```python
from build123d import *

# Parameters (mm, degrees)
F0_W     = 5
F0_H     = 4
F1_DEPTH = 6
F2_W     = 4
F2_H     = 2
F3_DEPTH = 25
F4_R     = 0.5
F5_DEPTH = 25
F6_R     = 1.25
F6_R_2   = 0.5
F7_DEPTH = 1
F8_R     = 1


with BuildPart() as f1:
    # F0 (on Top) → F1 (new body)
    with BuildSketch(Plane.XY):
        with Locations((2.5, 2)):
            Rectangle(F0_W, F0_H)
    extrude(amount=F1_DEPTH)

    # F2 (on face) → F3 (cut)
    with BuildSketch(Plane.XZ):
        with Locations((3, 3)):
            Rectangle(F2_W, F2_H)
    extrude(amount=-F3_DEPTH, mode=Mode.SUBTRACT)

    # F4 (on face) → F5 (cut)
    with BuildSketch(Plane.XY.offset(6)):
        with Locations((3, 2)):
            Circle(F4_R)
    extrude(amount=-F5_DEPTH, mode=Mode.SUBTRACT)

    # F6 (on face) → F7 (cut)
    with BuildSketch(Plane.XY.offset(6)):
        with Locations((3, 2)):
            Circle(F6_R)
        with Locations((3, 2)):
            Circle(F6_R_2, mode=Mode.SUBTRACT)
    extrude(amount=-F7_DEPTH, mode=Mode.SUBTRACT)

    # F8
    f8_edges = [f1.edges().sort_by_distance(p)[0] for p in [
        (5, 0, 1),
        (5, 0, 5),
        (5, 4, 5),
        (5, 4, 1),
    ]]
    fillet(f8_edges, radius=F8_R)


solid = f1.part
```
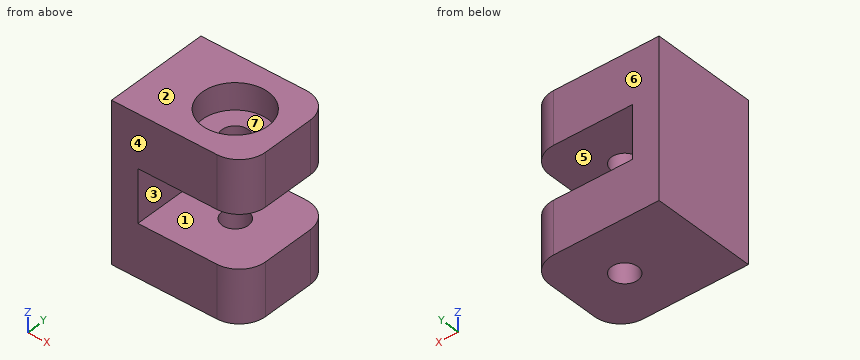
Input: part model. Units: mm. Frame: model coordinates. Face numbers are marked on the shaded views. A direction names the side the tool comes from. Coordinates: 2 decimals unless noted, no trailing zeros. Loops run counter-clockwise (first coordinate to the right, second up) from the corner with the lowest first, then second, coordinate; pieces in that order, holes last. Notation, with made-up numbers: (31, 4.5) -> (61, 4.5) arc R29 ccw to (61, 32.5) -> close; hole circle Ø1 at (-36.5, 35.25). An arc over 180 degrees is marked (long way). Use a Markdown table: item, result.
1) Access query for the marked faces 5, 6 and 7. Directions: +Z, -Z, +X, -X, +Y, -Y. A direction counts if a zero-diameter tool reaches every point of the face in a straight line with its end or side. Return the directions, or none.
Results found:
| item | result |
|---|---|
| face 5 | +X, +Y, -Y |
| face 6 | +Z, -Z, +X, -X, +Y |
| face 7 | +Z |
2) Pull-direction query (Z, two-part tool) for the marked faces 1, 2, 3 and 4; classes: released by +Z, released by -Z, zero draft, split by the parting line, or undercut.
Results found:
| item | result |
|---|---|
| face 1 | undercut |
| face 2 | released by +Z |
| face 3 | undercut |
| face 4 | zero draft |
3) Material intervals for line 1 along Y through (x, z) = (3, 0.55); line 2 along Z through (x, y) = (1.65, 0.8); line 3 along Z through (x, y) = (3.4, 1.25), sorted ascending. Write a range as from..to.
Results found:
| item | result |
|---|---|
| line 1 | y = 0..1.5, 2.5..4 |
| line 2 | z = 0..2, 4..6 |
| line 3 | z = 0..2, 4..5 |
4) Cut plane B-B (z = 4.8). Return the cut outline in (x, y).
Results found:
| item | result |
|---|---|
| outline | (0, 0) -> (4, 0) arc R1 ccw to (5, 1) -> (5, 3) arc R1 ccw to (4, 4) -> (0, 4) -> close; hole circle Ø1 at (3, 2) |
5) Cut plane C-C (x = 1.15). Return the cut outline in (y, z), then the cut area to 3 significant figures.
Results found:
| item | result |
|---|---|
| outline | (0, 0) -> (4, 0) -> (4, 2) -> (0, 2) -> close; (0, 4) -> (4, 4) -> (4, 6) -> (0, 6) -> close |
| area | 16.0 mm2 |
6) Cut plane A-A (y = 2). Return the cut outline in (x, z), then the cut area to 3 significant figures.
Results found:
| item | result |
|---|---|
| outline | (0, 0) -> (2.5, 0) -> (2.5, 2) -> (1, 2) -> (1, 4) -> (2.5, 4) -> (2.5, 5) -> (1.75, 5) -> (1.75, 6) -> (0, 6) -> close; (3.5, 0) -> (5, 0) -> (5, 2) -> (3.5, 2) -> close; (3.5, 4) -> (5, 4) -> (5, 6) -> (4.25, 6) -> (4.25, 5) -> (3.5, 5) -> close |
| area | 16.5 mm2 |
7) Cut plane D-D (x = 3). Return the cut outline in (y, z), then the cut area to 3 significant figures.
Results found:
| item | result |
|---|---|
| outline | (0, 0) -> (1.5, 0) -> (1.5, 2) -> (0, 2) -> close; (0, 4) -> (1.5, 4) -> (1.5, 5) -> (0.75, 5) -> (0.75, 6) -> (0, 6) -> close; (2.5, 0) -> (4, 0) -> (4, 2) -> (2.5, 2) -> close; (2.5, 4) -> (4, 4) -> (4, 6) -> (3.25, 6) -> (3.25, 5) -> (2.5, 5) -> close |
| area | 10.5 mm2 |
